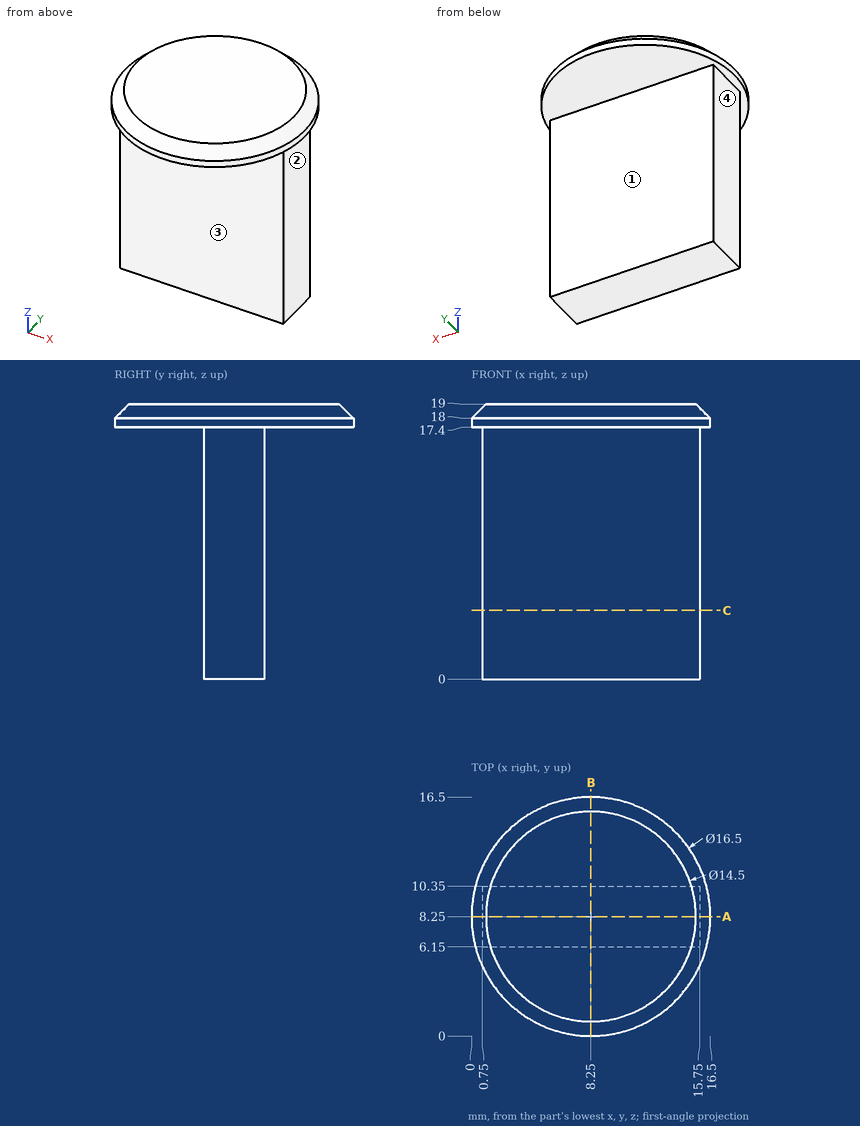
Verification items for this drawing (mm, ordinates from the low corner). A direction names the side the tool comes from. Give positions to 0.01 mm unless a question says otherwise; leave off trailing zeros. Write each loop counter-clockwise with the first axis right and the second up, starting at its lowest first coordinate (ties: lowest second). Pieces come first, ordered by that corner, then holes. Notation, with made-up numbers: (11, -7.75) - (34, -7.75) arc R16 cw to (34, 18.25) - close; hole circle Ø2 at (-31.75, -9). An arc over 180 degrees is marked (long way). Answer as CSV lines item,"result". Start each with the question number.
1. Depth check by flat-ended pin: pin 1 (1.3 mm diameter, centred on y = 8.5, z = 9, fed in from +X); pin 2 (6 mm diameter, centred on y = 14.5, z = 10, fed in from -X); pin 3 (3 mm diameter, centred on x = 4, z = 4, fed in from -Y); pin 4 (3.5 mm diameter, centred on y = 8.5, z = 13, fed in from -X). Enter the tip coordinate at first touch or a pass-through.
2. Sectioned sample at A-A (y = 8.25). Record the boundary of the cut face in (x, z), then the cut area to 3 significant figures.
3. Set-up check for the marked faces 1, 2, 3 and 4: record each of +Z, -Z, +X, -X, +Y, -Y from which the full face is reachable in a straight line by a thin tool's end or side.
4. Sectioned sample at B-B (x = 8.25). Record the boundary of the cut face in (y, z).
5. Sectioned sample at C-C (z = 4.75). Record the boundary of the cut face in (x, y).
6. Thickness scan on line 1 (Z direction, x = 4, y = 3.5); line 2 (Y direction, x = 4, z = 1.5); line 3 (X direction, y = 10, z = 4). Record the ranges inside material, lowest first.
Derived:
1,pin 1,"x = 15.75"
1,pin 2,"through"
1,pin 3,"y = 6.15"
1,pin 4,"x = 0.75"
2,outline,"(0, 17.4) - (0.75, 17.4) - (0.75, 0) - (15.75, 0) - (15.75, 17.4) - (16.5, 17.4) - (16.5, 18) - (15.5, 19) - (1, 19) - (0, 18) - close"
2,area,"286 mm²"
3,face 1,"-Z, +X, -X, +Y"
3,face 2,"-Z, +X, +Y, -Y"
3,face 3,"-Z, +X, -X, -Y"
3,face 4,"-Z, -X, +Y, -Y"
4,outline,"(0, 17.4) - (6.15, 17.4) - (6.15, 0) - (10.35, 0) - (10.35, 17.4) - (16.5, 17.4) - (16.5, 18) - (15.5, 19) - (1, 19) - (0, 18) - close"
5,outline,"(0.75, 6.15) - (15.75, 6.15) - (15.75, 10.35) - (0.75, 10.35) - close"
6,line 1,"17.4 to 19"
6,line 2,"6.15 to 10.35"
6,line 3,"0.75 to 15.75"
